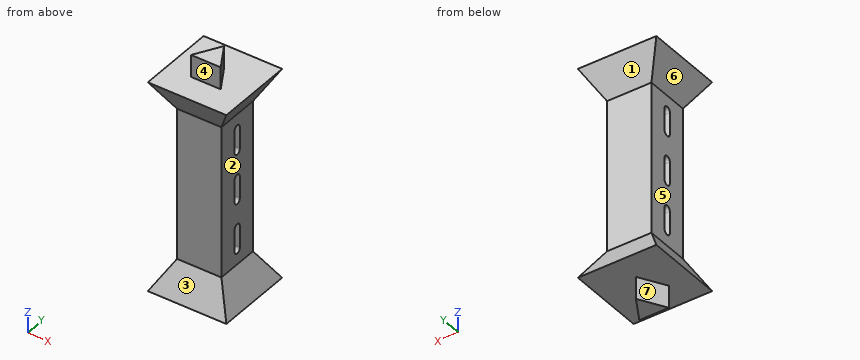
```python
from build123d import *

# Parameters (mm, degrees)
SKETCH1_W               = 3
SKETCH1_H               = 3
BOSS_EXTRUDE1_DEPTH     = 10.24
SKETCH2_W               = 3
SKETCH2_H               = 3
BOSS_EXTRUDE2_DEPTH     = 2
BOSS_EXTRUDE2_DRAFT     = -30
MIRROR1_COPY_1_SKETCH_W = 3
MIRROR1_COPY_1_SKETCH_H = 3
MIRROR1_COPY_1_DEPTH    = 2
MIRROR1_COPY_1_DRAFT    = -30
BOSS_EXTRUDE3_DEPTH     = 1.5
CUT_EXTRUDE1_REACH      = 16.598


with BuildPart() as part:
    # Sketch1 → Boss-Extrude1 (new body)
    with BuildSketch(Plane.XY):
        Rectangle(SKETCH1_W, SKETCH1_H)
    extrude(amount=BOSS_EXTRUDE1_DEPTH)


with BuildPart() as boss_extrude2_tool:
    # Sketch2 → Boss-Extrude2 (with draft: the straight prism first)
    with BuildSketch(Plane.XY.offset(10.24)):
        Rectangle(SKETCH2_W, SKETCH2_H)
    extrude(amount=BOSS_EXTRUDE2_DEPTH)
    # Boss-Extrude2: the draft: its side faces are tilted about the plane it starts from
    boss_extrude2_sides = [boss_extrude2_tool.faces().sort_by_distance(p)[0] for p in [
        (1.5, 0, 11.24),
        (0, 1.5, 11.24),
        (-1.5, 0, 11.24),
        (0, -1.5, 11.24),
    ]]
    draft(boss_extrude2_sides, Plane.XY.offset(10.24), BOSS_EXTRUDE2_DRAFT)


with BuildPart() as part_1:
    add(part.part)

    # Boss-Extrude2: add boss_extrude2_tool
    add(boss_extrude2_tool.part)


with BuildPart() as mirror1_copy_1_tool:
    # Mirror1 copy 1 sketch → Mirror1 copy 1 (with draft: the straight prism first)
    with BuildSketch(Plane(origin=(0, 0, 0), x_dir=(1, 0, 0), z_dir=(0, 0, -1))):
        Rectangle(MIRROR1_COPY_1_SKETCH_W, MIRROR1_COPY_1_SKETCH_H)
    extrude(amount=MIRROR1_COPY_1_DEPTH)
    # Mirror1 copy 1: the draft: its side faces are tilted about the plane it starts from
    mirror1_copy_1_sides = [mirror1_copy_1_tool.faces().sort_by_distance(p)[0] for p in [
        (1.5, 0, -1),
        (0, 1.5, -1),
        (-1.5, 0, -1),
        (0, -1.5, -1),
    ]]
    draft(mirror1_copy_1_sides, Plane(origin=(0, 0, 0), x_dir=(1, 0, 0), z_dir=(0, 0, -1)), MIRROR1_COPY_1_DRAFT)


with BuildPart() as part_2:
    add(part_1.part)

    # Mirror1 copy 1: add mirror1_copy_1_tool
    add(mirror1_copy_1_tool.part)

    # Sketch3 → Boss-Extrude3 (add)
    with BuildSketch(Plane.XY.offset(12.24)):
        Polygon((0, 0.866025404), (-1, -0.866025404), (1, -0.866025404), align=None)
    boss_extrude3 = extrude(amount=BOSS_EXTRUDE3_DEPTH)

    # Mirror2: Boss-Extrude3 across plane
    add(boss_extrude3.mirror(Plane.XY.offset(5.12)))

    # Sketch7 → Cut-Extrude1 (cut, up to next)
    with BuildSketch(Plane(origin=(1.5, 0, 0), x_dir=(0, 0, -1), z_dir=(1, 0, 0)), mode=Mode.PRIVATE) as cut_extrude1_sk1:
        with BuildLine():
            Line((-9.24, 0.25), (-7.74, 0.25))
            ThreePointArc((-7.74, 0.25), (-7.49, 0), (-7.74, -0.25))
            Line((-7.74, -0.25), (-9.24, -0.25))
            ThreePointArc((-9.24, -0.25), (-9.49, 0), (-9.24, 0.25))
        make_face()
    cut_extrude1_tool1 = extrude(cut_extrude1_sk1.sketch, amount=-CUT_EXTRUDE1_REACH, mode=Mode.PRIVATE) & part_2.part
    # Sketch7 → Cut-Extrude1 (cut, up to next)
    with BuildSketch(Plane(origin=(1.5, 0, 0), x_dir=(0, 0, -1), z_dir=(1, 0, 0)), mode=Mode.PRIVATE) as cut_extrude1_sk2:
        with BuildLine():
            Line((-5.87, 0.25), (-4.37, 0.25))
            ThreePointArc((-4.37, 0.25), (-4.12, 0), (-4.37, -0.25))
            Line((-4.37, -0.25), (-5.87, -0.25))
            ThreePointArc((-5.87, -0.25), (-6.12, 0), (-5.87, 0.25))
        make_face()
    cut_extrude1_tool2 = extrude(cut_extrude1_sk2.sketch, amount=-CUT_EXTRUDE1_REACH, mode=Mode.PRIVATE) & part_2.part
    # Sketch7 → Cut-Extrude1 (cut, up to next)
    with BuildSketch(Plane(origin=(1.5, 0, 0), x_dir=(0, 0, -1), z_dir=(1, 0, 0)), mode=Mode.PRIVATE) as cut_extrude1_sk3:
        with BuildLine():
            Line((-2.5, 0.25), (-1, 0.25))
            ThreePointArc((-1, 0.25), (-0.75, 0), (-1, -0.25))
            Line((-1, -0.25), (-2.5, -0.25))
            ThreePointArc((-2.5, -0.25), (-2.75, 0), (-2.5, 0.25))
        make_face()
    cut_extrude1_tool3 = extrude(cut_extrude1_sk3.sketch, amount=-CUT_EXTRUDE1_REACH, mode=Mode.PRIVATE) & part_2.part
    add(cut_extrude1_tool1.solids().sort_by_distance((1.5, 0, 8.49))[0], mode=Mode.SUBTRACT)
    add(cut_extrude1_tool2.solids().sort_by_distance((1.5, 0, 5.12))[0], mode=Mode.SUBTRACT)
    add(cut_extrude1_tool3.solids().sort_by_distance((1.5, 0, 1.75))[0], mode=Mode.SUBTRACT)


solid = part_2.part
```
Input: part model. Units: mm. Frame: model coordinates. Face numbers are marked on the shaded views. A direction names the side the tool comes from. Coordinates: 2 decimals unless noted, no trailing zeros. Write each loop counter-clockwise with the first axis right and the second up, starting at its lowest first coordinate (ties: lowest second). Pieces come first, ordered by that corner, then holes. Notation, with made-up numbers: M 18,-8 L 60,-8 A19 cw 60,21 Z; hole C -11.5,28.5 d8. An arc over 180 degrees is marked long. Use one line per item in the form item = value.
Q1. Section D-D (z = 3.5). Return loops of the section in (x, y), plus the area to 3 significant figures.
Answer below:
outline = M -1.5,-1.5 L 1.5,-1.5 L 1.5,1.5 L -1.5,1.5 Z
area = 9.00 mm²
Q2. Section C-C (y = 1.7). Return loops of the section in (x, z).
Answer below:
outline = M -2.65,-2 L 2.65,-2 L 1.7,-0.35 L -1.7,-0.35 Z; M -2.65,12.24 L -1.7,10.59 L 1.7,10.59 L 2.65,12.24 Z
Q3. Draft query along Z for the marked faces 5, 6 and 7. Return one class per face: released by +Z, released by -Z, zero draft, split by the parting line, or undercut.
Answer below:
face_5 = undercut
face_6 = undercut
face_7 = zero draft
Q4. Section A-A (y = 0). Return loops of the section in (x, z), plus the area to 3 significant figures.
Answer below:
outline = M -2.65,-2 L -0.5,-2 L -0.5,-3.5 L 0.5,-3.5 L 0.5,-2 L 2.65,-2 L 1.5,0 L 1.5,0.75 L -1.5,0.75 L -1.5,0 Z; M -2.65,12.24 L -1.5,10.24 L -1.5,9.49 L 1.5,9.49 L 1.5,10.24 L 2.65,12.24 L 0.5,12.24 L 0.5,13.74 L -0.5,13.74 L -0.5,12.24 Z; M -1.5,2.75 L 1.5,2.75 L 1.5,4.12 L -1.5,4.12 Z; M -1.5,6.12 L 1.5,6.12 L 1.5,7.49 L -1.5,7.49 Z
area = 32.3 mm²
Q5. Section B-B (x = 1.8). Return loops of the section in (y, z).
Answer below:
outline = M -2.65,-2 L 2.65,-2 L 1.8,-0.52 L -1.8,-0.52 Z; M -2.65,12.24 L -1.8,10.76 L 1.8,10.76 L 2.65,12.24 Z
Q6. First-contact query: pin 1 (1.5 mm diameter, centred on x = -2, z = 7.5, fed in from -Y); pin 2 (0.8 mm diameter, centred on x = 0.5, z = 5, fed in from +Y); pin 3 (0.5 mm diameter, centred on x = 0.5, z = -2.5, fed in from -Y). Flat tips, straight axial feed; report the tip coordinate or a pass-through.
Answer below:
pin_1 = -1.5
pin_2 = 1.5
pin_3 = -0.87
Q7. Material intervals for probe 1 along Y at (x, z) = (-0.2, 4.75); probe 2 along Y at (x, z) = (0.6, 0.25); probe 3 along Z at (x, y) = (1.25, 1.3), sorted ascending. Write a range as from..to.
Answer below:
probe_1 = -1.5..-0.25, 0.25..1.5
probe_2 = -1.5..1.5
probe_3 = -2..12.24
Q8. Set-up query: the marked faces 1, 2, 3 and 4. Return all of +Z, -Z, +X, -X, +Y, -Y with unobstructed straight access to the full face (end or side cutting, diameter ignored); none if empty.
Answer below:
face_1 = +X, -X, +Y
face_2 = +X, +Y, -Y
face_3 = +X, -X, -Y
face_4 = +Z, +X, -X, -Y
